Read the model definition and answer for the solid it produces. Units are mm, in the model's axes. Face numbers are marked on the shaded views. Give positions to 0.01 mm unless a question says otherwise; leave off trailing zeros. Write each loop counter-clockwise with the first axis right and the second up, starting at its lowest first coordinate (ties: lowest second). Pieces come first, ordered by that corner, then holes.
Autodesk Fusion 360 part; units mm, degrees
sketch "Sketch1" plane through (0, 0, 0) normal (0, 0, 1) x (1, 0, 0)
  circle A0 centre (0, 0) radius 127
  dimension "d1" = 254
extrude "Extrude1" add sketch "Sketch1" along normal blind 15.5
sketch "Sketch3" plane through (0, 0, 15.5) normal (0, 0, 1) x (-1, 0, 0)
  circle A0 centre (0, 0) radius 127
  circle A1 centre (0, 0) radius 25
  circle A2 centre (0, 0) radius 32.5
  circle A3 centre (0, 0) radius 42.5
  line L0 (4.375, -42.2742) -> (-4.375, -42.2742) construction
  line L1 (-4.375, -42.2742) -> (-4.375, -47.2742)
  line L2 (4.375, -42.2742) -> (4.375, -47.2742)
  line L3 (-4.375, -47.2742) -> (4.375, -47.2742) construction
  line L4 (0, -47.2742) -> (0, -73.7742) construction
  circle A4 centre (0, -73.7742) radius 27.5
  line L5 (-4.375, -42.2742) -> (-4.375, -32.2042)
  line L6 (4.375, -42.2742) -> (4.375, -32.2042)
  line L7 (-6.875, -41.9402) -> (-6.875, -31.7645)
  line L8 (-6.875, -41.9402) -> (6.875, -41.9402) construction
  line L9 (6.875, -41.9402) -> (6.875, -31.7645)
  line L10 (-34.423, 24.926) -> (-38.798, 17.3482) construction
  line L11 (-36.6105, 21.1371) -> (0, -42.2742) construction
  line L12 (34.423, 24.926) -> (38.798, 17.3482) construction
  line L13 (36.6105, 21.1371) -> (0, -42.2742) construction
  line L14 (-36.6105, 21.1371) -> (36.6105, 21.1371) construction
  line L15 (-38.798, 17.3482) -> (-30.0771, 12.3132)
  line L16 (-34.423, 24.926) -> (-25.7021, 19.891)
  line L17 (-34.423, 24.926) -> (-30.0929, 22.426)
  line L18 (-38.798, 17.3482) -> (-34.4679, 14.8482)
  circle A5 centre (-64.4531, 37.212) radius 27.5
  line L19 (-39.7588, 15.0162) -> (-32.8838, 26.924) construction
  line L20 (-39.7588, 15.0162) -> (-30.9464, 9.9283)
  line L21 (-32.8838, 26.924) -> (-24.0714, 21.8362)
  line L22 (34.423, 24.926) -> (30.0929, 22.426)
  line L23 (38.798, 17.3482) -> (34.4679, 14.8482)
  circle A6 centre (64.4531, 37.212) radius 27.5
  line L24 (34.423, 24.926) -> (25.7021, 19.891)
  line L25 (38.798, 17.3482) -> (30.0771, 12.3132)
  line L26 (32.8838, 26.924) -> (39.7588, 15.0162) construction
  line L27 (32.8838, 26.924) -> (24.0714, 21.8362)
  line L28 (39.7588, 15.0162) -> (30.9464, 9.9283)
  circle A7 centre (0, 0) radius 118.5
  line L29 (-38.798, 17.3482) -> (-43.1282, 19.8482)
  line L30 (-34.423, 24.926) -> (-38.7532, 27.426)
  line L31 (34.423, 24.926) -> (38.7532, 27.426)
  line L32 (38.798, 17.3482) -> (43.1282, 19.8482)
  line L33 (-43.1282, 19.8482) -> (-38.7532, 27.426) construction
  line L34 (38.7532, 27.426) -> (43.1282, 19.8482) construction
  dimension "d19" = 50
  dimension "d20" = 7.5
  dimension "d21" = 17.5
  dimension "d22" = 8.75
  dimension "d23" = 5
  dimension "d24" = 26.5
  dimension "d25" = 55
  dimension "d26" = 13.75
  dimension "d32" = 237
  dimension "d33" = 5
  dimension "d35" = 5
extrude "Extrude3" add sketch "Sketch3" along normal blind 4 contours A0 | A1 | A2 A3 L9 L28 | A2 A3 L22 L23 L24 L25 | A2 A3 L5 L6 | A3 A6 L31 L32 | A3 L1 L2 A4 | A2 A3 L21 L27 | A6 | A2 A3 L7 L20 | A4 | A2 A3 L15 L16 L17 L18 | A3 A5 L29 L30 | A5
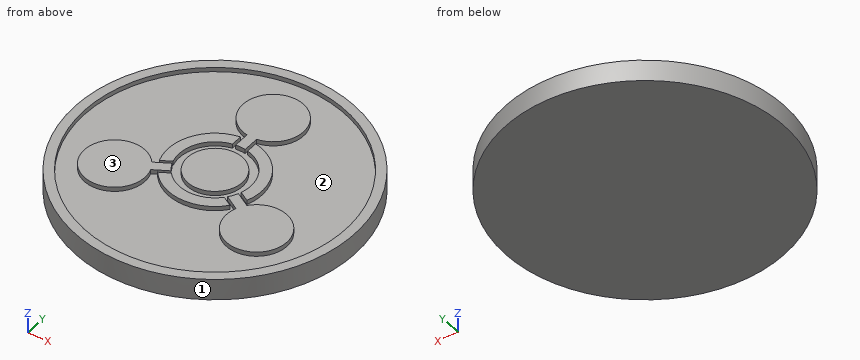
Item 1: Find the intervals of material crossed by line 1 along X through (y, z) = (0, 16.4); line 2 along Y through (x, z) = (-52, 16.25); line 3 along Y through (x, z) = (-66.5, 16), in increasing order.
Result set:
line 1: x = -127 to -118.5, -42.5 to -32.5, -25 to 25, 32.5 to 42.5, 118.5 to 127
line 2: y = -115.87 to -106.48, -61.73 to -12.69, 106.48 to 115.87
line 3: y = -108.2 to -98.08, -64.64 to -9.79, 98.08 to 108.2
Item 2: Section A-A (y = -37) is taken. Write down the section's boundary in (x, z).
Result set:
outline: (-121.49, 0) - (121.49, 0) - (121.49, 19.5) - (112.58, 19.5) - (112.58, 15.5) - (91.95, 15.5) - (91.95, 19.5) - (36.95, 19.5) - (36.95, 15.5) - (20.91, 15.5) - (20.91, 19.5) - (-20.91, 19.5) - (-20.91, 15.5) - (-36.95, 15.5) - (-36.95, 19.5) - (-91.95, 19.5) - (-91.95, 15.5) - (-112.58, 15.5) - (-112.58, 19.5) - (-121.49, 19.5) - close
Item 3: Section B-B (z = 12.5) is taken. Write down the section's boundary in (x, y), and give its area (3 significant figures).
Result set:
outline: circle Ø254 at (0, 0)
area: 50,700 mm2
Item 4: Determine the mould class of the marked faces 1, 2 and 3 for opening direction Y: pulls with the +Y half, pulls with the -Y half, needs draft (parallel to the pull), parting line crosses it, or undercut.
Result set:
face 1: parting line crosses it
face 2: undercut
face 3: needs draft
Item 5: Each of these flat-tipped pins is pushed along its axis until it touches: pin 1 Ø1 at (y, z) = (43, 7.5) entering from +X; pin 2 Ø3 at (y, z) = (34.5, 17) entering from +X; pin 3 Ø1 at (y, z) = (-84.5, 10.5) entering from +X. Where does it stop, or does it pass through?
Result set:
pin 1: stops at x = 119.68
pin 2: stops at x = 122.64
pin 3: stops at x = 95.25
